Geometry check sheet. Reference: the model listing, model coordinates, mm. Face numbers are marked on the shaded views. A direction names the side the tool comes from. Coordinates: 2 decimals unless noted, no trailing zeros. Loops run counter-clockwise (first coordinate to the right, second up) from the corner with the lowest first, then second, coordinate; pieces in that order, holes last.
from build123d import *

# Parameters (mm, degrees)
EXTRUDE_1_DEPTH     = 5
SKETCH_2_R          = 10
SKETCH_2_R_2        = 2
EXTRUDE_2_DEPTH     = 8
SHELL_1_OUTLINE_R   = 4.5
SHELL_1_DEPTH       = 2.5
SHELL_START         = 2.5
SHELL_1_2_OUTLINE_R = 4.5
SHELL_1_2_DEPTH     = 3
CUT_EXTRUDE_6_DEPTH = 2.5


with BuildPart() as part:
    # ｽｹｯﾁ1 → ﾎﾞｽ - 押し出し1 (new body)
    with BuildSketch(Plane.XY):
        Polygon((-15, -77.5), (15, -77.5), (17.362836016, -64.5), (23.688654544, -61.502664525), (26, 0.497335475), (33.120827994, 6.001316642), (30.14, 57.5), (17, 74.5), (-17, 74.5), (-30.14, 57.5), (-33.120827994, 6.001316642), (-26, 0.497335475), (-23.688654544, -61.502664525), (-17.362836016, -64.5), align=None)
    extrude(amount=EXTRUDE_1_DEPTH)

    # ｽｹｯﾁ2 → ﾎﾞｽ - 押し出し2 (add)
    # profile 1 of 8: a face of its own
    with BuildSketch(Plane(origin=(0, 0, 0), x_dir=(-1, 0, 0), z_dir=(0, 0, -1))):
        with BuildLine():
            Line((-32.382872215, 18.750710787), (-31.011292455, 42.446996487))
            Line((-31.011292455, 42.446996487), (-46.596716305, 51.215377732))
            ThreePointArc((-46.596716305, 51.215377732), (-42.867710705, 47.548126536), (-41.5, 42.5))
            ThreePointArc((-41.5, 42.5), (-46.653423142, 33.752960915), (-56.802138552, 34.021360559))
            Line((-56.802138552, 34.021360559), (-32.382872215, 18.750710787))
        make_face()
    # profile 2 of 8: a face of its own
    with BuildSketch(Plane(origin=(0, 0, 0), x_dir=(-1, 0, 0), z_dir=(0, 0, -1))):
        with Locations((-51.5, 42.5)):
            Circle(SKETCH_2_R)
        with Locations((-51.5, 42.5)):
            Circle(SKETCH_2_R_2, mode=Mode.SUBTRACT)
    # profile 3 of 8: a face of its own
    with BuildSketch(Plane(origin=(0, 0, 0), x_dir=(-1, 0, 0), z_dir=(0, 0, -1))):
        with Locations((51.5, 42.5)):
            Circle(SKETCH_2_R)
        with Locations((51.5, 42.5)):
            Circle(SKETCH_2_R_2, mode=Mode.SUBTRACT)
    # profile 4 of 8: a face of its own
    with BuildSketch(Plane(origin=(0, 0, 0), x_dir=(-1, 0, 0), z_dir=(0, 0, -1))):
        with Locations((51.5, -82.5)):
            Circle(SKETCH_2_R)
        with Locations((51.5, -82.5)):
            Circle(SKETCH_2_R_2, mode=Mode.SUBTRACT)
    # profile 5 of 8: a face of its own
    with BuildSketch(Plane(origin=(0, 0, 0), x_dir=(-1, 0, 0), z_dir=(0, 0, -1))):
        with BuildLine():
            Line((16.09996425, -71.448147417), (46.056282089, -90.888440577))
            ThreePointArc((46.056282089, -90.888440577), (43.199925585, -76.922476831), (57.20989431, -74.290425896))
            Line((57.20989431, -74.290425896), (24.071173493, -51.241898524))
            Line((24.071173493, -51.241898524), (23.688654544, -61.502664525))
            Line((23.688654544, -61.502664525), (17.362836016, -64.5))
            Line((17.362836016, -64.5), (16.09996425, -71.448147417))
        make_face()
    # profile 6 of 8: a face of its own
    with BuildSketch(Plane(origin=(0, 0, 0), x_dir=(-1, 0, 0), z_dir=(0, 0, -1))):
        with BuildLine():
            ThreePointArc((56.802138552, 34.021360559), (42.900678635, 37.395916139), (46.596716305, 51.215377732))
            Line((46.596716305, 51.215377732), (31.011292455, 42.446996487))
            Line((31.011292455, 42.446996487), (32.382872215, 18.750710787))
            Line((32.382872215, 18.750710787), (56.802138552, 34.021360559))
        make_face()
    # profile 7 of 8: a face of its own
    with BuildSketch(Plane(origin=(0, 0, 0), x_dir=(-1, 0, 0), z_dir=(0, 0, -1))):
        with BuildLine():
            Line((-46.056282089, -90.888440577), (-16.09996425, -71.448147417))
            Line((-16.09996425, -71.448147417), (-17.362836016, -64.5))
            Line((-17.362836016, -64.5), (-23.688654544, -61.502664525))
            Line((-23.688654544, -61.502664525), (-24.071173493, -51.241898524))
            Line((-24.071173493, -51.241898524), (-57.20989431, -74.290425896))
            ThreePointArc((-57.20989431, -74.290425896), (-46.868528479, -73.637186025), (-41.5, -82.5))
            ThreePointArc((-41.5, -82.5), (-42.712589144, -87.272987581), (-46.056282089, -90.888440577))
        make_face()
    # profile 8 of 8: a face of its own
    with BuildSketch(Plane(origin=(0, 0, 0), x_dir=(-1, 0, 0), z_dir=(0, 0, -1))):
        with Locations((-51.5, -82.5)):
            Circle(SKETCH_2_R)
        with Locations((-51.5, -82.5)):
            Circle(SKETCH_2_R_2, mode=Mode.SUBTRACT)
    extrude(amount=-EXTRUDE_2_DEPTH)

    # ｼｪﾙ1: read off the stored shape, not the designer's step
    # ｼｪﾙ1 outline → ｼｪﾙ1 (cut)
    with BuildSketch(Plane.XY):
        with BuildLine():
            Line((21.522008123, -52.514136891), (23.545326343, 1.75976204))
            Line((23.545326343, 1.75976204), (30.548821684, 7.173051968))
            Line((30.548821684, 7.173051968), (29.801456877, 20.085002485))
            Line((29.801456877, 20.085002485), (55.476603914, 36.141020419))
            ThreePointArc((55.476603914, 36.141020419), (57.949491024, 46.328062896), (47.822537229, 49.036533299))
            Line((47.822537229, 49.036533299), (28.746880144, 38.304541956))
            Line((28.746880144, 38.304541956), (27.688881042, 56.583208435))
            Line((27.688881042, 56.583208435), (15.772608032, 72))
            Line((15.772608032, 72), (-15.772608032, 72))
            Line((-15.772608032, 72), (-27.688881042, 56.583208435))
            Line((-27.688881042, 56.583208435), (-28.746880144, 38.304541956))
            Line((-28.746880144, 38.304541956), (-47.822537229, 49.036533299))
            ThreePointArc((-47.822537229, 49.036533299), (-57.949491024, 46.328062896), (-55.476603914, 36.141020419))
            Line((-55.476603914, 36.141020419), (-29.801456877, 20.085002485))
            Line((-29.801456877, 20.085002485), (-30.548821684, 7.173051968))
            Line((-30.548821684, 7.173051968), (-23.545326343, 1.75976204))
            Line((-23.545326343, 1.75976204), (-21.522008123, -52.514136891))
            Line((-21.522008123, -52.514136891), (-55.782420733, -76.342819422))
            ThreePointArc((-55.782420733, -76.342819422), (-57.725055812, -86.683142377), (-47.417211567, -88.791330433))
            Line((-47.417211567, -88.791330433), (-14.311630395, -67.307308042))
            Line((-14.311630395, -67.307308042), (-12.913432732, -75))
            Line((-12.913432732, -75), (12.913432732, -75))
            Line((12.913432732, -75), (14.311630395, -67.307308042))
            Line((14.311630395, -67.307308042), (47.417211567, -88.791330433))
            ThreePointArc((47.417211567, -88.791330433), (57.725055812, -86.683142377), (55.782420733, -76.342819422))
            Line((55.782420733, -76.342819422), (21.522008123, -52.514136891))
        make_face()
        with Locations((51.5, -82.5)):
            Circle(SHELL_1_OUTLINE_R, mode=Mode.SUBTRACT)
        with Locations((-51.5, -82.5)):
            Circle(SHELL_1_OUTLINE_R, mode=Mode.SUBTRACT)
        with Locations((-51.5, 42.5)):
            Circle(SHELL_1_OUTLINE_R, mode=Mode.SUBTRACT)
        with Locations((51.5, 42.5)):
            Circle(SHELL_1_OUTLINE_R, mode=Mode.SUBTRACT)
    extrude(amount=SHELL_1_DEPTH, mode=Mode.SUBTRACT)

    # Shell 1 2 outline → Shell 1 2 (cut)
    # profile 1 of 4: a face of its own
    with BuildSketch(Plane.XY.offset(SHELL_START)):
        with BuildLine():
            Line((55.782420733, -76.342819422), (26.399026656, -55.906183789))
            Line((26.399026656, -55.906183789), (26.130390005, -63.112147889))
            Line((26.130390005, -63.112147889), (19.593043591, -66.209710715))
            Line((19.593043591, -66.209710715), (18.857369821, -70.257286993))
            Line((18.857369821, -70.257286993), (47.417211567, -88.791330433))
            ThreePointArc((47.417211567, -88.791330433), (57.725055812, -86.683142377), (55.782420733, -76.342819422))
        make_face()
        with Locations((51.5, -82.5)):
            Circle(SHELL_1_2_OUTLINE_R, mode=Mode.SUBTRACT)
    # profile 2 of 4: a face of its own
    with BuildSketch(Plane.XY.offset(SHELL_START)):
        with BuildLine():
            Line((33.597298428, 41.033394063), (34.634873185, 23.10759156))
            Line((34.634873185, 23.10759156), (55.476603914, 36.141020419))
            ThreePointArc((55.476603914, 36.141020419), (57.949491024, 46.328062896), (47.822537229, 49.036533299))
            Line((47.822537229, 49.036533299), (33.597298428, 41.033394063))
        make_face()
        with Locations((51.5, 42.5)):
            Circle(SHELL_1_2_OUTLINE_R, mode=Mode.SUBTRACT)
    # profile 3 of 4: a face of its own
    with BuildSketch(Plane.XY.offset(SHELL_START)):
        with BuildLine():
            Line((-47.417211567, -88.791330433), (-18.857369821, -70.257286993))
            Line((-18.857369821, -70.257286993), (-19.593043591, -66.209710715))
            Line((-19.593043591, -66.209710715), (-26.130390005, -63.112147889))
            Line((-26.130390005, -63.112147889), (-26.399026656, -55.90618379))
            Line((-26.399026656, -55.90618379), (-55.782420733, -76.342819422))
            ThreePointArc((-55.782420733, -76.342819422), (-57.725055812, -86.683142377), (-47.417211567, -88.791330433))
        make_face()
        with Locations((-51.5, -82.5)):
            Circle(SHELL_1_2_OUTLINE_R, mode=Mode.SUBTRACT)
    # profile 4 of 4: a face of its own
    with BuildSketch(Plane.XY.offset(SHELL_START)):
        with BuildLine():
            Line((-34.634873185, 23.10759156), (-33.597298428, 41.033394063))
            Line((-33.597298428, 41.033394063), (-47.822537229, 49.036533299))
            ThreePointArc((-47.822537229, 49.036533299), (-57.949491024, 46.328062896), (-55.476603914, 36.141020419))
            Line((-55.476603914, 36.141020419), (-34.634873185, 23.10759156))
        make_face()
        with Locations((-51.5, 42.5)):
            Circle(SHELL_1_2_OUTLINE_R, mode=Mode.SUBTRACT)
    extrude(amount=SHELL_1_2_DEPTH, mode=Mode.SUBTRACT)

    # ｽｹｯﾁ5 → ｶｯﾄ - 押し出し6 (cut)
    with BuildSketch(Plane(origin=(0, 0, 0), x_dir=(-1, 0, 0), z_dir=(0, 0, -1))):
        Polygon((-38.80400438, 46.831187109), (-38.80400438, 43.962694111), (-39.472839378, 23.184439628), (-51.319731768, 2.127093459), (-84.265468017, 28.099065241), (-81.185505749, 33.573566869), (-64.091586556, 65.569805047), (-41.966326194, 51.733717696), align=None)
        Polygon((-39.472839378, -51.723167443), (-24.731165472, -89.760648138), (-36.427967097, -116.261009638), (-70.745334213, -107.593739558), (-74.01113331, -73.736521524), align=None)
        Polygon((70.745334213, -107.593739558), (74.01113331, -73.736521524), (39.472839378, -51.723167443), (24.731165472, -89.760648138), (36.427967097, -116.261009638), align=None)
        Polygon((64.091586556, 65.569805047), (41.966326194, 51.733717696), (38.80400438, 46.831187109), (38.80400438, 43.962694111), (39.472839378, 23.184439628), (51.319731768, 2.127093459), (84.265468017, 28.099065241), (81.185505749, 33.573566869), align=None)
    extrude(amount=-CUT_EXTRUDE_6_DEPTH, mode=Mode.SUBTRACT)


solid = part.part
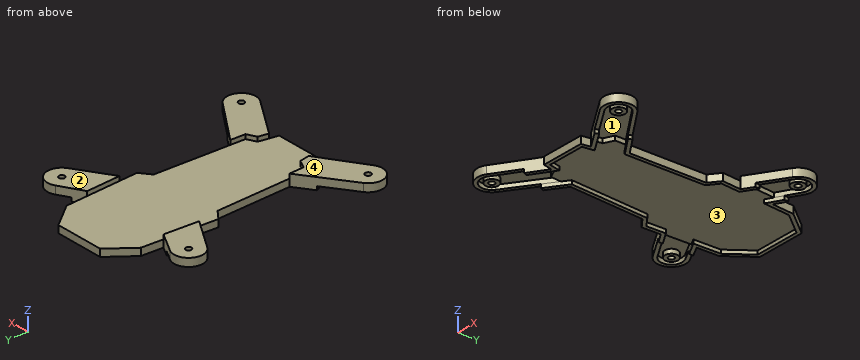
1) Depth check by flat-ended pin: pin 1 (10 mm diameter, centred on x = -53.5, y = 43, fed in from -Z); pin 2 (10 mm diameter, centred on x = -40, y = -73, fed in from -Z); pin 3 (1.2 mm diameter, centred on x = 0, z = 1.5, fed in from -Y). Enter the tip coordinate at first touch or a pass-through.
Data:
pin 1: stops at z = 2.5
pin 2: stops at z = 5.5
pin 3: stops at y = -77.5
2) Access from +Z, -Z, +X, -X, +Y, -Y to the whole of each face (thin tool, end or side, straight path). Record for the marked faces 1 and 2.
Data:
face 1: -Z
face 2: +Z, +X, -X, +Y, -Y
3) Section check B-B on x = -2.5. Record the cut outline in (y, z).
Data:
outline: (-77.5, 0) - (-75, 0) - (-75, 2.5) - (72, 2.5) - (72, 0) - (74.5, 0) - (74.5, 5) - (-77.5, 5) - close
4) Section check C-C on y = -82.5. Count the separate pieces of the cut face and the enclosed holes in it, and give its area (3 significant figures).
Data:
separate pieces: 4
enclosed holes: 0
area: 194 mm2
5) Section check A-A on z = 6.75. Record the cut outline in (x, y), and give its area (3 significant figures).
Data:
outline: (-57.21, -74.29) arc R10 ccw to (-46.06, -90.89) - (-16.1, -71.45) - (-17.36, -64.5) - (-23.69, -61.5) - (-24.07, -51.24) - close; (-56.8, 34.02) - (-32.38, 18.75) - (-31.01, 42.45) - (-46.6, 51.22) arc R10 ccw to start; (16.1, -71.45) - (46.06, -90.89) arc R10 ccw to (57.21, -74.29) - (24.07, -51.24) - (23.69, -61.5) - (17.36, -64.5) - close; (31.01, 42.45) - (32.38, 18.75) - (56.8, 34.02) arc R10 ccw to (46.6, 51.22) - close; hole circle Ø4 at (-51.5, -82.5); hole circle Ø4 at (-51.5, 42.5); hole circle Ø4 at (51.5, -82.5); hole circle Ø4 at (51.5, 42.5)
area: 3,050 mm2
6) Mould release check, pull along X, two halves, no side actions. Record for the marked faces 3 and 4: +X half, -X half, draft (parallel to the pull), parting line (faces both ways), or undercut.
Data:
face 3: undercut
face 4: draft
7) Material ranges on probe 1 along Y at (x, z) = (-41.5, 3.75); probe 2 along X at (y, z) = (-76, 3); probe 3 along Z at (x, y) = (-15.5, -27), recorded low to high.
Data:
probe 1: y = -87.93 to -84.95, -66.41 to -63.36, 24.45 to 27.4, 45.48 to 48.35
probe 2: x = -59.1 to -55.29, -27.71 to -23.11, -15.27 to 15.27, 23.11 to 27.71, 55.29 to 59.1
probe 3: z = 2.5 to 5
